Geometry check sheet. Reference: the model listing, model coordinates, mm. Face numbers are marked on the shaded views. Coordinates: 2 decimals unless noted, no trailing zeros. Order: outer loops, then holes, each group sorted by start corner. A loop starts at its lowest first (then second) coordinate and runs counter-clockwise, first axis right, second up.
```python
from build123d import *

# Parameters (mm, degrees)
SKETCH1_W           = 23.5
SKETCH1_H           = 13
BOSS_EXTRUDE1_DEPTH = 4
SKETCH4_W           = 12
SKETCH4_H           = 3.5
BOSS_EXTRUDE3_DEPTH = 12
SKETCH5_R           = 0.8
CUT_EXTRUDE2_DEPTH  = 3
SKETCH6_R           = 1.3
CUT_EXTRUDE3_DEPTH  = 4


with BuildPart() as part:
    # Sketch1 → Boss-Extrude1 (new body)
    with BuildSketch(Plane.XY):
        with BuildLine():
            Line((24.860467777, 7.362362669), (-10.139532223, 7.362362669))
            ThreePointArc((-10.139532223, 7.362362669), (-12.294111981, 0.751764817), (-17.178188495, -4.196771785))
            ThreePointArc((-17.178188495, -4.196771785), (-15.407020853, -9.874958003), (-10.139532223, -12.637637331))
            Line((-10.139532223, -12.637637331), (24.860467777, -12.637637331))
            ThreePointArc((24.860467777, -12.637637331), (54.82087059, -8.185603487), (82.192202879, 4.785769252))
            ThreePointArc((82.192202879, 4.785769252), (82.614789286, 5.070273598), (83.035963889, 5.356863806))
            ThreePointArc((83.035963889, 5.356863806), (82.132298227, 10.279823625), (77.956940726, 7.519654292))
            ThreePointArc((77.956940726, 7.519654292), (51.420959061, 3.304188228), (24.860467777, 7.362362669))
        make_face()
        with Locations((7.360467777, -2.637637331)):
            Rectangle(SKETCH1_W, SKETCH1_H, mode=Mode.SUBTRACT)
    extrude(amount=BOSS_EXTRUDE1_DEPTH)

    # Sketch4 → Boss-Extrude3 (add)
    with BuildSketch(Plane(origin=(0, 0, 0), x_dir=(-1, 0, 0), z_dir=(0, 0, -1))):
        with Locations((-2.110467777, -10.887637331)):
            Rectangle(SKETCH4_W, SKETCH4_H)
    extrude(amount=BOSS_EXTRUDE3_DEPTH)

    # Sketch5 → Cut-Extrude2 (cut)
    with BuildSketch(Plane(origin=(0, 0, -12), x_dir=(-1, 0, 0), z_dir=(0, 0, -1))):
        with Locations((0.889532223, -10.887637331)):
            Circle(SKETCH5_R)
        with Locations((-5.110467777, -10.887637331)):
            Circle(SKETCH5_R)
    extrude(amount=-CUT_EXTRUDE2_DEPTH, mode=Mode.SUBTRACT)

    # Sketch6 → Cut-Extrude3 (cut)
    with BuildSketch(Plane.XY.offset(4)):
        with Locations((21.210467777, -2.637637331)):
            Circle(SKETCH6_R)
        with Locations((-6.489532223, -2.637637331)):
            Circle(SKETCH6_R)
    extrude(amount=-CUT_EXTRUDE3_DEPTH, mode=Mode.SUBTRACT)


solid = part.part
```
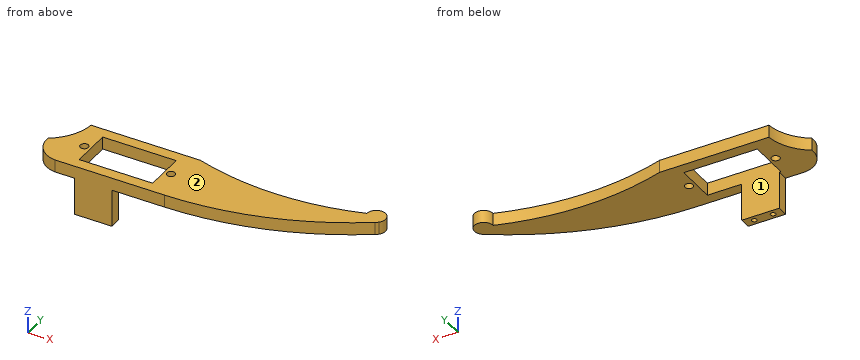
Item 1: Release check for a two-part mould opening along X. For the marked faces 1 and 2 record: pulls with the +X half, pulls with the -X half, needs draft (parallel to the pull), parting line crosses it, or undercut.
Item 2: Depth check by flat-ended pin: P1, Ø3, axis at x = 21.21, y = -2.64, coming from the -Z side; P2, Ø1.2, axis at y = -3, z = 2.5, coming from the +X side; P3, Ø2, axis at x = -6.49, y = -2.64, coming from the -Z side; P4, Ø1.8, axis at y = -10, z = -7.5, coming from the +X side. Enter the tip coordinate at first touch or a pass-through.
Item 3: Sectioned sample at B-B (y = 0). Record the cut outline in (x, z).
Item 4: Sectioned sample at A-A (x = 13.5). Record the cut outline in (y, z).
Item 5: Sectioned sample at D-D (z = -2.5). Record the cut outline in (x, y).
Item 6: Thickness scan on line 1 along Y through (x, z) = (12, 3.25); line 2 along X through (y, z) = (-3.75, 3.25); line 3 along Z through (x, y) = (-5.5, -9.25). Record the ranges inside material, lowest first.
Item 7: Sectioned sample at C-C (z = 2.5). Record the cut outline in (x, y), and give its area (3 significant figures).
Geometry check:
1. face 1: undercut
1. face 2: needs draft
2. P1: stops at z = 0
2. P2: stops at x = 69.64
2. P3: passes through
2. P4: stops at x = 8.11
3. outline: (-12.78, 0) - (-4.39, 0) - (-4.39, 4) - (-12.78, 4) - close; (19.11, 0) - (74.3, 0) - (74.3, 4) - (19.11, 4) - close
4. outline: (-12.64, 0) - (-9.14, 0) - (-9.14, 4) - (-12.64, 4) - close; (3.86, 0) - (7.36, 0) - (7.36, 4) - (3.86, 4) - close
5. outline: (-3.89, -12.64) - (8.11, -12.64) - (8.11, -9.14) - (-3.89, -9.14) - close
6. line 1: y = -12.64 to -9.14, 3.86 to 7.36
6. line 2: x = -16.51 to -7.16, -5.82 to -4.39, 19.11 to 20.54, 21.88 to 66.72
6. line 3: z = 0 to 4
7. outline: (-17.18, -4.2) arc R7.77 ccw to (-10.14, -12.64) - (24.86, -12.64) arc R103.04 ccw to (82.19, 4.79) arc R103.04 ccw to (83.04, 5.36) arc R3 ccw (long way) to (77.96, 7.52) arc R87.26 cw to (24.86, 7.36) - (-10.14, 7.36) arc R15.13 cw to start; hole circle Ø2.6 at (-6.49, -2.64); hole (-4.39, -9.14) - (19.11, -9.14) - (19.11, 3.86) - (-4.39, 3.86) - close; hole circle Ø2.6 at (21.21, -2.64)
7. area: 1,160 mm2
